The listing builds one solid part. Answer for the finished solid, in the listing's coordinates (mm). Face numbers are marked on the shaded views. A direction names the side the tool comes from. Round coordinates to 2 decimals unless told otherwise and drop trailing zeros. Loops run counter-clockwise (first coordinate to the right, second up) from the corner with the lowest first, then second, coordinate; pieces in that order, holes last. Notation, with made-up numbers: (11, 38.5) -> (36, 38.5) arc R31 ccw to (36, 77.5) -> close; hole circle Ø3 at (62, -29.5). An arc over 180 degrees is marked (long way). Use a Markdown table: item, result. Add a question column.
Q1. Section B-B on z = 8 is taken. Give the vertices of the cut face in (x, y), then the cut area to 3 significant figures.
Q2. Section D-D on y = 8.75 is taken. Give the vertices of the cut face in (x, z).
Q3. Section A-A on y = 1.6 is taken. Give the vertices of the cut face in (x, z).
Q4. Given pin 1 Ø3.5 at (y, z) = (2, 4.5) entering from -X; pin 2 Ø4 at (x, z) = (5, 5.5) entering from +Y, each flat-ended and moving along its own axis, determine where each tip first touches the part or whether it passes through.
Q5. For a pull along X with two mould halves and no side action, classify the marked faces 4, 5, 6 and 7 as released by +X, released by -X, zero draft, split by the parting line, or undercut.
Q6. Section C-C on x = 4 is taken. Give the vertices of the cut face in (y, z).
Q7. Which of the six approach directions +Z, -Z, +X, -X, +Y, -Y give full straight-line access (tool end or side, diameter ignored) to the marked faces 1, 2 and 3?
Q8. Consider line 1 (Y direction, x = 6.5, z = 10.25); line 2 (Y direction, x = 4.75, z = 6); line 3 (X direction, y = 3.5, z = 12). Determine where each line is inside the solid, lowest interval first.
from build123d import *

# Parameters (mm, degrees)
SKETCH1_W           = 8
SKETCH1_H           = 3.2
BOSS_EXTRUDE1_DEPTH = 16
SKETCH2_W           = 4.8
SKETCH2_H           = 12.8
CUT_EXTRUDE1_DEPTH  = 1.8
SKETCH3_R           = 2.4
BOSS_EXTRUDE2_DEPTH = 1.8
SKETCH4_R           = 1.6
BOSS_EXTRUDE3_DEPTH = 1.8
SWEEP1_PROFILE_R    = 1.5


with BuildPart() as part:
    # Sketch1 → Boss-Extrude1 (new body)
    with BuildSketch(Plane.XY):
        with Locations((4, 1.6)):
            Rectangle(SKETCH1_W, SKETCH1_H)
    extrude(amount=BOSS_EXTRUDE1_DEPTH)

    # Sketch2 → Cut-Extrude1 (cut)
    with BuildSketch(Plane.XZ):
        with Locations((4, 8)):
            Rectangle(SKETCH2_W, SKETCH2_H)
    extrude(amount=-CUT_EXTRUDE1_DEPTH, mode=Mode.SUBTRACT)

    # Sketch3 → Boss-Extrude2 (add)
    with BuildSketch(Plane(origin=(0, 3.2, 0), x_dir=(1, 0, 0), z_dir=(0, 1, 0))):
        with Locations(Location((4, -4, 0), (0, 0, 90))):
            Circle(SKETCH3_R)
        with Locations(Location((4, -12, 0), (0, 0, 90))):
            Circle(SKETCH3_R)
    extrude(amount=BOSS_EXTRUDE2_DEPTH)

    # Sketch4 → Boss-Extrude3 (add)
    with BuildSketch(Plane.XZ.offset(-1.8)):
        with Locations(Location((4, 8, 0), (0, 0, 270))):
            Circle(SKETCH4_R)
    extrude(amount=BOSS_EXTRUDE3_DEPTH)

    # Sweep1: sweep along a path in Sketch6
    with BuildLine(Plane.XY.offset(8)) as sweep1_path:
        Line((0, 1.6), (-4, 1.6))
        Line((-4, 1.6), (-4, 9.6))
    # Sweep1 profile (on start of the path) → Sweep1 (sweep)
    with BuildSketch(Plane(origin=(0, 1.6, 8), x_dir=(0, -1, 0), z_dir=(-1, 0, 0))):
        Circle(SWEEP1_PROFILE_R)
    sweep(path=sweep1_path.line, transition=Transition.RIGHT)


solid = part.part
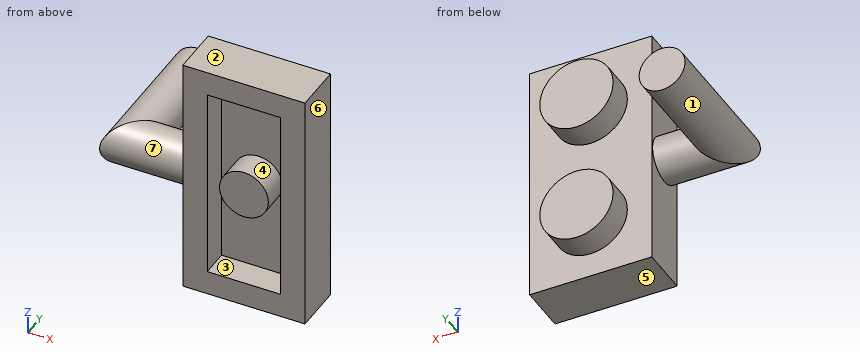
Checked values:
| question | item | result |
|---|---|---|
| 1 | outline | (-5.5, 0.1) -> (0, 0.1) -> (0, 0) -> (1.6, 0) -> (1.6, 1.8) -> (2.4, 1.8) -> (2.4, 0) -> (5.6, 0) -> (5.6, 1.8) -> (6.4, 1.8) -> (6.4, 0) -> (8, 0) -> (8, 3.2) -> (0, 3.2) -> (0, 3.1) -> (-2.5, 3.1) -> (-2.5, 9.6) -> (-5.5, 9.6) -> close |
| 1 | area | 58.7 mm2 |
| 2 | outline | circle Ø3 at (-4, 8) |
| 3 | outline | (-4, 6.5) -> (0, 6.5) -> (0, 0) -> (8, 0) -> (8, 16) -> (0, 16) -> (0, 9.5) -> (-4, 9.5) arc R1.5 ccw to start; circle Ø3.2 at (4, 8); hole (1.6, 1.6) -> (6.4, 1.6) -> (6.4, 14.4) -> (1.6, 14.4) -> close |
| 4 | pin 1 | stops at x = 0 |
| 4 | pin 2 | stops at y = 5 |
| 5 | face 4 | undercut |
| 5 | face 5 | zero draft |
| 5 | face 6 | released by +X |
| 5 | face 7 | undercut |
| 6 | outline | (0, 0) -> (3.2, 0) -> (3.2, 1.6) -> (5, 1.6) -> (5, 6.4) -> (3.2, 6.4) -> (3.2, 9.6) -> (5, 9.6) -> (5, 14.4) -> (3.2, 14.4) -> (3.2, 16) -> (0, 16) -> (0, 14.4) -> (1.8, 14.4) -> (1.8, 9.6) -> (0, 9.6) -> (0, 6.4) -> (1.8, 6.4) -> (1.8, 1.6) -> (0, 1.6) -> close |
| 7 | face 1 | +Y |
| 7 | face 2 | +Z, +X, -X, +Y, -Y |
| 7 | face 3 | -Y |
| 8 | line 1 | y = 0 to 3.2 |
| 8 | line 2 | y = 1.8 to 5 |
| 8 | line 3 | x = 1.6 to 6.4 |
